Part print with two shaded views. Sizes in mm from the minimum x, y, z corner. Round coordinates to 2 decimals unless told otherwise and drop trailing zeros. Write each loop counter-clockwise with the first axis right and the second up, starting at its lowest first coordinate (ties: lowest second). Pieces come first, ordered by that corner, then holes. Notation, with made-up numbers: (-19.5, 64) -> (28.5, 64) arc R27 ccw to (28.5, 96) -> close; hole circle Ø7 at (80, 42). An arc over 180 degrees is marked (long way). Return JSON: item names as keys, results as strings.
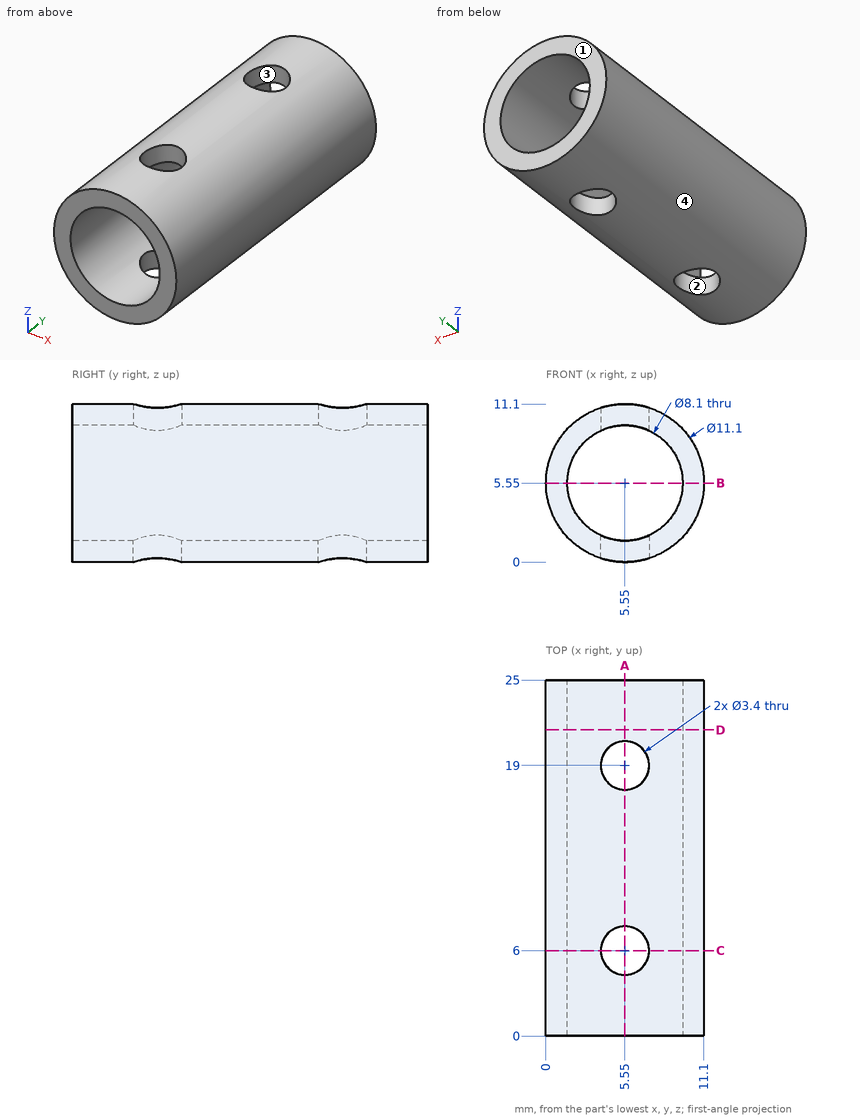
Q1. Two-plate mould, pull along X, no slides. Class the marked faces 1, 2, 3 and 4: +X half, -X half, draft (parallel to the pull), parting line (faces both ways), or undercut.
Verdict:
{"face 1": "draft", "face 2": "undercut", "face 3": "undercut", "face 4": "parting line"}
Q2. Wall check: L1, parallel to Y at x = 5.55, z = 9.7; L2, parallel to Z at x = 5.55, y = 11.5. Give the ranges that are in metal, low to high.
Verdict:
{"L1": "y = 0 to 4.3, 7.7 to 17.3, 20.7 to 25", "L2": "z = 0 to 1.5, 9.6 to 11.1"}
Q3. Saw through at A-A on x = 5.55. List the corners of the cut face in (y, z).
Verdict:
{"outline": "(0, 0) -> (4.3, 0) -> (4.3, 1.5) -> (0, 1.5) -> close; (0, 9.6) -> (4.3, 9.6) -> (4.3, 11.1) -> (0, 11.1) -> close; (7.7, 0) -> (17.3, 0) -> (17.3, 1.5) -> (7.7, 1.5) -> close; (7.7, 9.6) -> (17.3, 9.6) -> (17.3, 11.1) -> (7.7, 11.1) -> close; (20.7, 0) -> (25, 0) -> (25, 1.5) -> (20.7, 1.5) -> close; (20.7, 9.6) -> (25, 9.6) -> (25, 11.1) -> (20.7, 11.1) -> close"}
Q4. Saw through at C-C on y = 6. List the corners of the cut face in (x, z), then the cut area to 3 significant figures.
Verdict:
{"outline": "(3.85, 0.27) -> (3.85, 1.87) arc R4.05 cw to (3.85, 9.23) -> (3.85, 10.83) arc R5.55 ccw to start; (7.25, 0.27) arc R5.55 ccw to (7.25, 10.83) -> (7.25, 9.23) arc R4.05 cw to (7.25, 1.87) -> close", "area": "34.8 mm²"}
Q5. Saw through at B-B on z = 5.55. List the corners of the cut face in (x, y).
Verdict:
{"outline": "(0, 0) -> (1.5, 0) -> (1.5, 25) -> (0, 25) -> close; (9.6, 0) -> (11.1, 0) -> (11.1, 25) -> (9.6, 25) -> close"}
Q6. Saw through at D-D on y = 21.5. List the corners of the cut face in (x, z).
Verdict:
{"outline": "circle Ø11.1 at (5.55, 5.55); hole circle Ø8.1 at (5.55, 5.55)"}
Q7. Pin check, flat tips, straight feed: pin 1 Ø4.5 at (x, y) = (5.55, 6) entering from -Z; pin 2 Ø4 at (y, z) = (3.5, 2.5) entering from -X; pin 3 Ø3 at (x, z) = (4.5, 3.5) entering from -Y. Stop position of each tip, or through.
Verdict:
{"pin 1": "stops at z = 0", "pin 2": "stops at x = 0.1", "pin 3": "passes through"}
